Design review of the part built by this model. Coordinates are the model's own, in mm. A direction names the side the tool comes from. Give positions to 0.01 mm unless a question says otherwise; leave off trailing zeros. Write each loop counter-clockwise with the first axis right and the second up, starting at its lowest first coordinate (ties: lowest second). Pieces come first, ordered by that corner, then holes. Notation, with made-up numbers: M -15,84.5 L 9,84.5 A9 ccw 9,89.5 Z; hole C 11.5,62.25 d1. An arc over 180 degrees is marked long. Answer in a Markdown table with one row per item.
```python
from build123d import *

# Parameters (mm, degrees)
BOSS_EXTRUDE1_REACH     = 44
SKETCH4_R               = 2.5
CUT_EXTRUDE1_DEPTH      = 10
CUT_EXTRUDE1_DEPTH_BACK = 10


with BuildPart() as part:
    # Sketch1 → Revolve1 (revolve)
    with BuildSketch(Plane.XY):
        with BuildLine():
            Line((-8.485281374, 3), (-7.2, 3))
            Line((-7.2, 3), (-7.2, -3))
            Line((-7.2, -3), (-8.485281374, -3))
            ThreePointArc((-8.485281374, -3), (-9, 0), (-8.485281374, 3))
        make_face()
    revolve(axis=Axis((0, -4.387716131, 0), (0, 1, 0)))

    # Sketch4 → Boss-Extrude1 (add, up to next)
    with BuildSketch(Plane.XY.offset(33), mode=Mode.PRIVATE) as boss_extrude1_sk1:
        Circle(SKETCH4_R)
    boss_extrude1_tool1 = extrude(boss_extrude1_sk1.sketch, amount=-BOSS_EXTRUDE1_REACH, mode=Mode.PRIVATE) - part.part
    add(boss_extrude1_tool1.solids().sort_by_distance((0, 0, 33))[0])

    # Sketch5 → Revolve2 (revolve)
    with BuildSketch(Plane(origin=(0, 0, 0), x_dir=(1, 0, 0), z_dir=(0, 1, 0))):
        with BuildLine():
            Line((0, -7.8), (0, -15.691021161))
            Line((0, -15.691021161), (-7.372368399, -5.162187927))
            ThreePointArc((-7.372368399, -5.162187927), (-8.583452557, -2.706352196), (-9, 0))
            Line((-9, 0), (-7.8, 0))
            ThreePointArc((-7.8, 0), (-5.515432893, -5.515432893), (0, -7.8))
        make_face()
    revolve(axis=Axis((0, 0, 0), (0, 0, 1)))

    # Sketch6 → Cut-Extrude1 (cut, two sides)
    with BuildSketch(Plane.ZY) as cut_extrude1_sk:
        Polygon((0, 3), (11.40657714, 3), (12.120651144, 2.5), (12, 3), (12, 13), (0, 13), align=None)
        Polygon((0, -3), (11.40657714, -3), (12.120651144, -2.5), (12, -3), (12, -13), (0, -13), align=None)
    extrude(amount=CUT_EXTRUDE1_DEPTH, mode=Mode.SUBTRACT)
    extrude(cut_extrude1_sk.sketch, amount=-CUT_EXTRUDE1_DEPTH_BACK, mode=Mode.SUBTRACT)


solid = part.part
```
1) Insertion check: P1, Ø8, axis at x = 2, z = 19, coming from the -Y side; P2, Ø1, axis at x = -1.5, y = 1, coming from the -Z side; P3, Ø2, axis at y = 0, z = 22.5, coming from the -X side. Each pin has a flat end and moves straight along its axis. Give the tip position at first contact, or say it passes through.
Geometry says:
| item | result |
|---|---|
| P1 | y = -2.5 |
| P2 | z = -8.91 |
| P3 | x = -2.5 |
2) Add section C-C (y = 0). Write out the cut boundary in (x, z).
Geometry says:
| item | result |
|---|---|
| outline | M -7.37,5.16 A9 ccw long 7.37,5.16 L 2.5,12.12 L 2.5,33 L -2.5,33 L -2.5,12.12 Z; hole C 0,0 d14.4 |
3) Add section B-B (z = 0). Write out the cut boundary in (x, y).
Geometry says:
| item | result |
|---|---|
| outline | M -8.49,-3 L -7.2,-3 L -7.2,3 L -8.49,3 A9 ccw Z; M 7.2,-3 L 8.49,-3 A9 ccw 8.49,3 L 7.2,3 Z |
4) To check wall thickness, follow probe 1 along Z at (x, y) = (0, 0.1); probe 2 along X at (y, z) = (0.35, 0); probe 3 along Z at (x, y) = (-2.75, 0). State the ranges of each line that lie inside material, in increasing order. Write a range as [from, to].
Geometry says:
| item | result |
|---|---|
| probe 1 | [-9, -7.2], [7.2, 33] |
| probe 2 | [-8.99, -7.2], [7.2, 8.99] |
| probe 3 | [-8.57, -6.65], [6.65, 11.76] |
5) Add section A-A (x = 0). Write out the cut boundary in (y, z), and give its area (3 significant figures).
Geometry says:
| item | result |
|---|---|
| outline | M -3,-8.49 A9 ccw 3,-8.49 L 3,-7.2 L -3,-7.2 Z; M -3,7.2 L 3,7.2 L 3,11.41 L 2.5,12.12 L 2.5,33 L -2.5,33 L -2.5,12.12 L -3,11.41 Z |
| area | 143 mm^2 |
6) Add section D-D (z = 21). Write out the cut boundary in (x, y), and give its area (3 significant figures).
Geometry says:
| item | result |
|---|---|
| outline | C 0,0 d5 |
| area | 19.6 mm^2 |
7) The part is to be moulded in two halves that separate along Z. For faces 3 (the face through (-1.2, 3, 7.3)), 4 (the face through (-6.87, -0.04, 2.16)), 5 (the face through (-3.091, 1.282, 10.912)), say which applies: released by +Z, released by -Z, zero draft, split by the parting line, or undercut.
Geometry says:
| item | result |
|---|---|
| face 3 | zero draft |
| face 4 | undercut |
| face 5 | released by +Z |
8) For faces 1 (the face through (-0.54, -2.44, 22.71)), 2 (the face through (0, 0, 33)), list the 3-axis set-ups (+Z, -Z, +X, -X, +Y, -Y) from which the entire face can be reached by the end or side of a thin tool; tool diameter is ignored.
Geometry says:
| item | result |
|---|---|
| face 1 | +Z |
| face 2 | +Z, +X, -X, +Y, -Y |
